The drawing under review shows one solid part. Ordinate dimensions are in mm from its lowest x, y, z. A direction names the side the tool comes from. Coordinates: 2 decimals unless noted, no trailing zeros. Loops run counter-clockwise (first coordinate to the right, second up) from the corner with the lowest first, then second, coordinate; pieces in that order, holes last. Notation, with made-up numbers: (44, 32.25) - (61, 32.25) arc R8 cw to (61, 40.25) - close; hole circle Ø1 at (24, 87.5). An arc over 180 degrees is marked (long way). Answer as a JSON object with one key per item and string values. Group by question number.
Item 1: Tool access review of the marked faces 4, 5, 6 and 7: name each direction out of +Z, -Z, +X, -X, +Y, -Y from which nothing blocks a thin tool from reaching the whole face with its end or side.
Item 2: We need section B-B (z = 14.5). Give the boundary of the cut face in (x, y).
Item 3: To check wall thickness, follow line 1 (X direction, y = 16.75, z = 80.5); line 2 (X direction, y = 18.75, z = 30); line 3 (Z direction, x = 18.5, y = 14.5). State the ranges of each line that lie inside material, in increasing order.
Item 4: Mouldability with a two-part tool opening along X and no side actions: class the marked faces 1, 2 and 3 as released by +X, released by -X, zero draft, split by the parting line, or undercut.
Item 5: We need section D-D (x = 76). Give the boundary of the cut face in (y, z) (1 decimal).
Item 6: We need section C-C (x = 17.5). Give the boundary of the cut face in (y, z).
Item 7: Clearance check with flat-ended pins moving along their axes: pin 1 (7.5 mm diameter, centred on y = 9, z = 80, fed in from +X); pin 2 (10 mm diameter, centred on x = 16, y = 19.5, fed in from -Z); pin 3 (4 mm diameter, centred on x = 78, y = 8, fed in from +Z) (1 decimal). State where each tip first meets the part, or that it passes through.
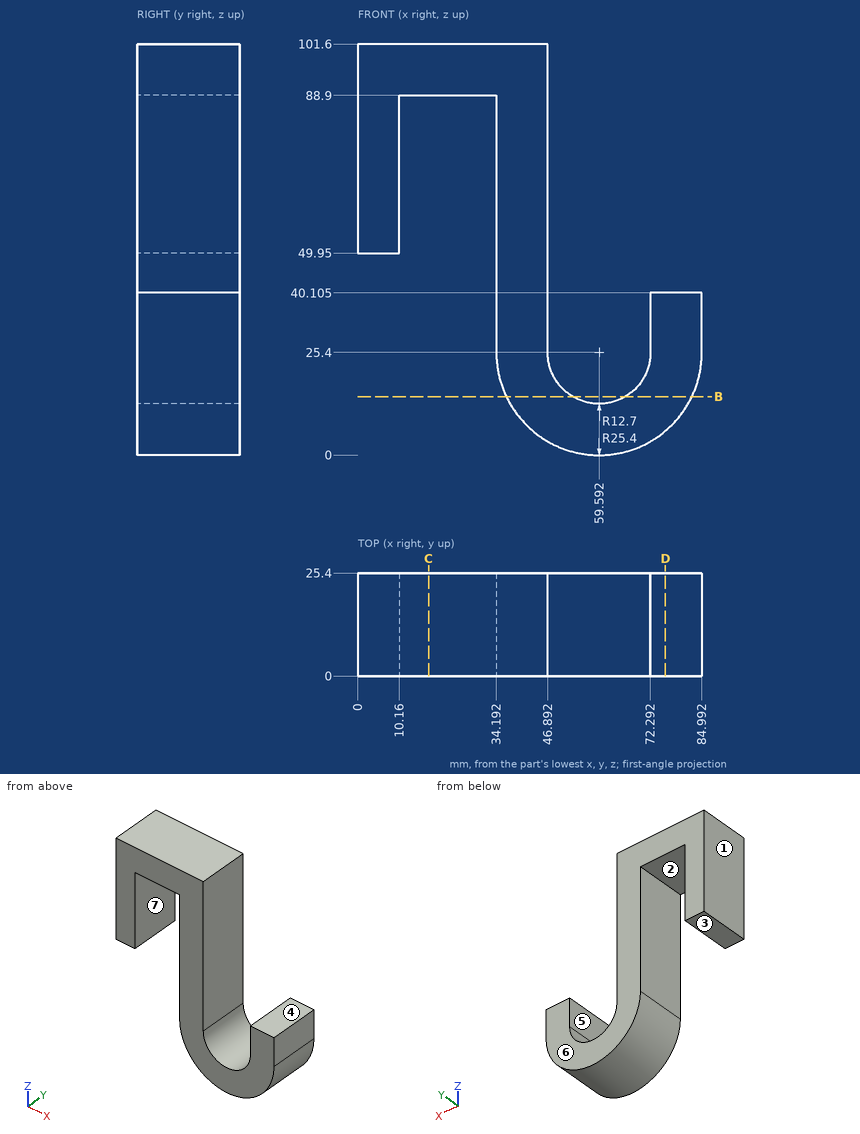
Check sheet entries:
{
 "1": {"face 4": "+Z, +X, +Y, -Y", "face 5": "+Z, +Y, -Y", "face 6": "+Z, -Z, +X, -X, +Y", "face 7": "-Z, +Y, -Y"},
 "2": {"outline": "(36.65, 0) - (53.07, 0) - (53.07, 25.4) - (36.65, 25.4) - close; (66.11, 0) - (82.53, 0) - (82.53, 25.4) - (66.11, 25.4) - close"},
 "3": {"line 1": "x = 0 to 10.16, 34.19 to 46.89", "line 2": "x = 34.19 to 46.89, 72.29 to 84.99", "line 3": "z = 88.9 to 101.6"},
 "4": {"face 1": "released by -X", "face 2": "undercut", "face 3": "zero draft"},
 "5": {"outline": "(0, 6) - (25.4, 6) - (25.4, 40.1) - (0, 40.1) - close"},
 "6": {"outline": "(0, 88.9) - (25.4, 88.9) - (25.4, 101.6) - (0, 101.6) - close"},
 "7": {"pin 1": "stops at x = 46.89", "pin 2": "stops at z = 88.9", "pin 3": "stops at z = 40.1"}
}
